Here's the drawing with two shaded views (mm, measured from the low corner). I have some questions. Coordinates: 2 decimals unless noted, no trailing zeros. Write each loop counter-clockwise with the first axis right and the second up, starting at its lowest first coordinate (ties: lowest second). Pieces come first, ordered by that corner, then holes.
Item 1: I'm going to push flat-ended pins straight in: pin 1 Ø1.5 at (x, y) = (39.5, 13.5) entering from -Z; pin 2 Ø2.5 at (x, y) = (41.2, 3.4) entering from +Z; pin 3 Ø2 at (y, z) = (14, 9) entering from +X; pin 4 Ø1.2 at (x, y) = (4, 17.6) entering from -Z. Where does each tip first touch, or does it pass through?
Item 2: If we section it at B-B (x = 11.6): Please give me the cut outline in (y, z), then the cut area to 3 significant figures.
Item 3: If we section it at C-C (x = 21): Please give me the cut outline in (y, z), then the cut area to 3 significant figures.
Item 4: If I drill on line 1 (X direction, y = 10.25, z = 3.75) (1 decimal); line 2 (Y direction, x = 32.5, z = 3.75) (1 decimal); line 3 (X direction, y = 7.5, z = 9.5) (1 decimal), over which ranges is the centre line in solid material (lowest first)?
Item 5: We'd pull the mould along Y, two halves only. Please class the marked faces 1, 2 and 3: +Y half, -Y half, draft (parallel to the pull), parting line (faces both ways), or undercut.
Item 6: If we section it at A-A (z = 6.75): Please give me the cut outline in (x, y).
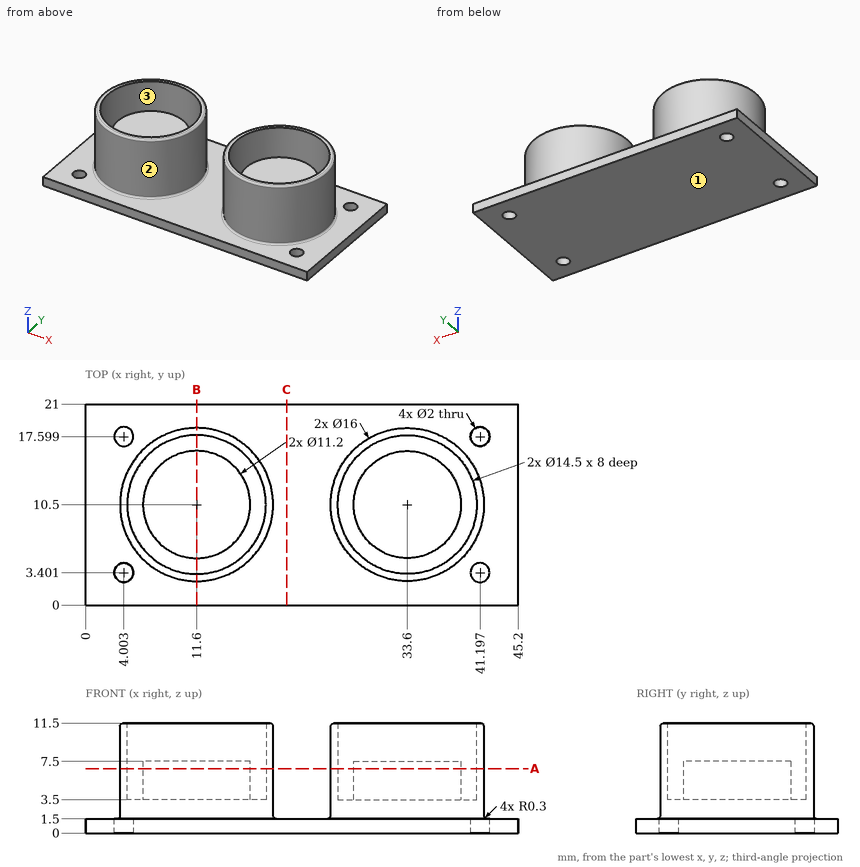
Answer list:
1. pin 1: stops at z = 0
1. pin 2: stops at z = 1.5
1. pin 3: stops at x = 41.2
1. pin 4: passes through
2. outline: (0, 0) - (21, 0) - (21, 1.5) - (18.8, 1.5) arc R0.3 cw to (18.5, 1.8) - (18.5, 11.2) arc R0.3 ccw to (18.2, 11.5) - (17.75, 11.5) - (17.75, 3.5) - (16.1, 3.5) - (16.1, 7.5) - (4.9, 7.5) - (4.9, 3.5) - (3.25, 3.5) - (3.25, 11.5) - (2.8, 11.5) arc R0.3 ccw to (2.5, 11.2) - (2.5, 1.8) arc R0.3 cw to (2.2, 1.5) - (0, 1.5) - close
2. area: 120 mm2
3. outline: (0, 0) - (21, 0) - (21, 1.5) - (0, 1.5) - close
3. area: 31.5 mm2
4. line 1: x = 3.6 to 4.4, 6 to 17.2, 18.8 to 19.6, 25.6 to 26.4, 28 to 39.2, 40.8 to 41.6
4. line 2: y = 2.6 to 3.3, 5 to 16, 17.7 to 18.4
4. line 3: x = 4.2 to 5, 18.2 to 19, 26.2 to 27, 40.2 to 41
5. face 1: draft
5. face 2: parting line
5. face 3: undercut
6. outline: circle Ø16 at (11.6, 10.5); circle Ø11.2 at (11.6, 10.5); circle Ø16 at (33.6, 10.5); circle Ø11.2 at (33.6, 10.5); hole circle Ø14.5 at (11.6, 10.5); hole circle Ø14.5 at (33.6, 10.5)
